Read the model definition and answer for the solid it produces. Units are mm, in the model's axes. Face numbers are marked on the shaded views. A direction names the side the tool comes from. Coordinates: 2 decimals unless noted, no trailing zeros. Loops run counter-clockwise (first coordinate to the right, second up) from the corner with the lowest first, then second, coordinate; pieces in that order, holes last. Notation, with made-up numbers: M 28,-25 L 78,-25 A11 cw 78,-12 Z; hole C -30.75,84.5 d5. An arc over 180 degrees is marked long. Use one line per item in the form item = value. Start each with the question number.
1. The part is cut by section C-C (x = 223). Give the vertices of the cut face in (y, z).
2. Flat-ended cylindrical pins translate along their axes: pin 1 (16.5 mm diameter, centred on x = 398.5, z = -177.5, fed in from -Y); pin 2 (10 mm diameter, centred on y = 358, z = -124.5, fed in from -X); pin 3 (4.5 mm diameter, centred on x = -48, z = 375.5, fed in from +Y). Find the tip coordinate at first contact, or state that the pin passes through.
3. Find the intervals of material crossed by probe 1 along X at (y, z) = (204, 77); probe 2 along Z at (x, y) = (301.5, 238); probe 3 along Z at (x, y) = (-101.5, 416), in increasing order. Write a range as [from, to].
4. A tool of negligible diameter and unlimited length cuts with its end or side. For the marked faces 1, 2, 3, 4 and 5, from which of +Z, -Z, +X, -X, +Y, -Y can it reach the whole face along a straight path? Write none if from no direction.
5. For a pull along X with two mould halves and no side action, classify the marked faces 6, 7 and 8 as released by +X, released by -X, zero draft, split by the parting line, or undercut.
6. The part is cut by section D-D (z = -222). Give the vertices of the cut face in (x, y).
7. The part is cut by section B-B (y = 96.5). Give the vertices of the cut face in (x, z), plus the area to 3 significant figures.
8. The part is cut by section A-A (z = 100). Give the vertices of the cut face in (x, y).
from build123d import *

# Parameters (mm, degrees)
F0_W      = 435
F0_H      = 465
F1_DEPTH  = 15
F3_DEPTH  = 480
F4_DEPTH  = 3
F5_W      = 15
F5_H      = 720
F6_DEPTH  = 483
F8_DEPTH  = 5
F9_R      = 25
F10_DEPTH = 5
F12_DEPTH = 18
F13_W     = 15
F13_H     = 240
F14_DEPTH = 330
F15_W     = 15
F15_H     = 240
F16_DEPTH = 330


with BuildPart() as f1:
    # F0 (on Top) → F1 (new body)
    with BuildSketch(Plane.XY):
        with Locations((173.112164, 216.248717)):
            Rectangle(F0_W, F0_H)
    extrude(amount=F1_DEPTH)

    # F2 (on face) → F3 (join)
    with BuildSketch(Plane.XZ.offset(16.251283)):
        Polygon((-59.387836, 195), (-59.387836, 0), (-59.387836, -525), (-44.387836, -525), (-44.387836, 195), align=None)
    extrude(amount=-F3_DEPTH)

    # F2 (on face) → F4 (join)
    with BuildSketch(Plane.XZ.offset(16.251283)):
        Polygon((-59.387836, 195), (-59.387836, 0), (-59.387836, -525), (-44.387836, -525), (-44.387836, 195), align=None)
    extrude(amount=F4_DEPTH)

    # F5 (on face) → F6 (join)
    with BuildSketch(Plane.XZ.offset(19.251283)):
        with Locations((398.112164, -165)):
            Rectangle(F5_W, F5_H)
    extrude(amount=-F6_DEPTH)

    # F7 (on face) → F8 (join)
    with BuildSketch(Plane(origin=(0, 448.748717, 0), x_dir=(-1, 0, 0), z_dir=(0, 1, 0))):
        Polygon((-390.612164, 195), (-390.612164, 15), (-390.612164, -525), (44.387836, -525), (44.387836, 195), align=None)
    extrude(amount=F8_DEPTH)

    # F9 (on face) → F10 (cut)
    with BuildSketch(Plane(origin=(0, 453.748717, 0), x_dir=(-1, 0, 0), z_dir=(0, 1, 0))):
        with Locations((-173.112164, 100)):
            Circle(F9_R)
    extrude(amount=-F10_DEPTH, mode=Mode.SUBTRACT)

    # F11 (on face) → F12 (join)
    with BuildSketch(Plane.XY.offset(195)):
        with BuildLine():
            Line((-750.387836, -89.251283), (414.612164, -89.251283))
            ThreePointArc((414.612164, -89.251283), (425.218766, -84.857884), (429.612164, -74.251283))
            Line((429.612164, -74.251283), (429.612164, 500.748717))
            Line((429.612164, 500.748717), (-765.387836, 500.748717))
            Line((-765.387836, 500.748717), (-765.387836, -74.251283))
            ThreePointArc((-765.387836, -74.251283), (-760.994438, -84.857884), (-750.387836, -89.251283))
        make_face()
    extrude(amount=F12_DEPTH)

    # F13 (on face) → F14 (join)
    with BuildSketch(Plane.XY.offset(213)):
        with Locations((409.112164, 373.748717)):
            Rectangle(F13_W, F13_H)
    extrude(amount=F14_DEPTH)

    # F15 (on face) → F16 (join)
    with BuildSketch(Plane.XY.offset(213)):
        with Locations((-45.887836, 373.748717)):
            Rectangle(F15_W, F15_H)
    extrude(amount=F16_DEPTH)


solid = f1.part
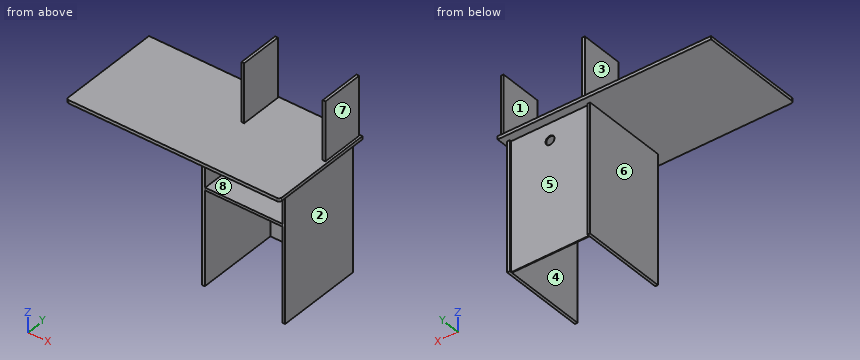
Computed values:
q1.outline = M -89.25,195 L 448.75,195 L 448.75,15 L -16.25,15 L -16.25,0 L 448.75,0 L 448.75,-525 L 453.75,-525 L 453.75,195 L 500.75,195 L 500.75,213 L -89.25,213 Z
q2.pin_1 = -19.25
q2.pin_2 = -59.39
q2.pin_3 = 493.75
q3.probe_1 = [-59.39, -44.39], [390.61, 405.61]
q3.probe_2 = [0, 15], [195, 213]
q3.probe_3 = [195, 213]
q4.face_1 = +Z, +Y, -Y
q4.face_2 = -Z, +X, +Y, -Y
q4.face_3 = +Z, -X, +Y, -Y
q4.face_4 = -Y
q4.face_5 = -Z, +Y
q5.face_6 = released by -X
q5.face_7 = released by +X
q5.face_8 = undercut
q6.outline = M -59.39,-19.25 L -44.39,-19.25 L -44.39,448.75 L 390.61,448.75 L 390.61,-19.25 L 405.61,-19.25 L 405.61,463.75 L 390.61,463.75 L 390.61,453.75 L -44.39,453.75 L -44.39,463.75 L -59.39,463.75 Z
q7.outline = M -765.39,195 L -59.39,195 L -59.39,-525 L -44.39,-525 L -44.39,0 L 390.61,0 L 390.61,-525 L 405.61,-525 L 405.61,195 L 429.61,195 L 429.61,213 L -765.39,213 Z; hole M -44.39,15 L 390.61,15 L 390.61,195 L -44.39,195 Z
q7.area = 49,600 mm²
q8.outline = M -59.39,-19.25 L -44.39,-19.25 L -44.39,448.75 L 148.11,448.75 L 148.11,453.75 L -44.39,453.75 L -44.39,463.75 L -59.39,463.75 Z; M 198.11,448.75 L 390.61,448.75 L 390.61,-19.25 L 405.61,-19.25 L 405.61,463.75 L 390.61,463.75 L 390.61,453.75 L 198.11,453.75 Z
